Geometry: final body of the model. Coordinates: model frame, mm. Face numbers are marked on the shaded views. A direction names the side the tool comes from. Coordinates: 2 decimals unless noted, no trailing zeros. Loops run counter-clockwise (first coordinate to the right, second up) from the corner with the lowest first, then second, coordinate; pieces in that order, holes last. Notation, with made-up numbers: (-17.5, -0.75) -> (-7.5, -0.75) arc R21 ccw to (-7.5, 8.25) -> close; hole circle Ø11 at (55.5, -40). An arc over 180 degrees is marked (long way). One line per item, written item: value. Start each with the question number.
from build123d import *

# Parameters (mm, degrees)
SKETCH1_W           = 180
SKETCH1_H           = 200
BOSS_EXTRUDE1_DEPTH = 12.5
SKETCH2_W           = 85
SKETCH2_H           = 55
CUT_EXTRUDE1_DEPTH  = 1.5
SKETCH3_W           = 105
SKETCH3_H           = 35
CUT_EXTRUDE2_DEPTH  = 1.5
SKETCH4_W           = 180
SKETCH4_H           = 200
CUT_EXTRUDE3_DEPTH  = 4.5
SKETCH5_W           = 180
SKETCH5_H           = 200
CUT_EXTRUDE4_DEPTH  = 3
SKETCH7_W           = 85
SKETCH7_H           = 55
BOSS_EXTRUDE2_DEPTH = 1.5
SKETCH8_W           = 50
SKETCH8_H           = 50
CUT_EXTRUDE5_DEPTH  = 1.5
SKETCH9_W           = 66
SKETCH9_H           = 36
CUT_EXTRUDE6_DEPTH  = 1.5
SKETCH11_W          = 80
SKETCH11_H          = 40
SKETCH11_W_2        = 97
SKETCH11_H_2        = 20
CUT_EXTRUDE9_DEPTH  = 1.5
SKETCH15_R          = 1.35
CUT_EXTRUDE11_DEPTH = 135.629120178
SKETCH16_R          = 1.75
CUT_EXTRUDE12_DEPTH = 5


with BuildPart() as part:
    # Sketch1 → Boss-Extrude1 (new body)
    with BuildSketch(Plane(origin=(0, 0, 0), x_dir=(1, 0, 0), z_dir=(0, 1, 0))):
        Rectangle(SKETCH1_W, SKETCH1_H)
    extrude(amount=BOSS_EXTRUDE1_DEPTH)

    # Sketch2 → Cut-Extrude1 (cut)
    with BuildSketch(Plane(origin=(0, 12.5, 0), x_dir=(1, 0, 0), z_dir=(0, 1, 0))):
        Rectangle(SKETCH2_W, SKETCH2_H)
    extrude(amount=-CUT_EXTRUDE1_DEPTH, mode=Mode.SUBTRACT)

    # Sketch3 → Cut-Extrude2 (cut)
    with BuildSketch(Plane(origin=(0, 12.5, 0), x_dir=(1, 0, 0), z_dir=(0, 1, 0))):
        with Locations((0, 67.5)):
            Rectangle(SKETCH3_W, SKETCH3_H)
    extrude(amount=-CUT_EXTRUDE2_DEPTH, mode=Mode.SUBTRACT)

    # Sketch4 → Cut-Extrude3 (cut)
    with BuildSketch(Plane.XZ):
        Rectangle(SKETCH4_W, SKETCH4_H)
    extrude(amount=-CUT_EXTRUDE3_DEPTH, mode=Mode.SUBTRACT)

    # Sketch5 → Cut-Extrude4 (cut)
    with BuildSketch(Plane.XZ.offset(-4.5)):
        Rectangle(SKETCH5_W, SKETCH5_H)
    extrude(amount=-CUT_EXTRUDE4_DEPTH, mode=Mode.SUBTRACT)

    # Sketch7 → Boss-Extrude2 (add)
    with BuildSketch(Plane(origin=(0, 11, 0), x_dir=(1, 0, 0), z_dir=(0, 1, 0))):
        Rectangle(SKETCH7_W, SKETCH7_H)
    extrude(amount=BOSS_EXTRUDE2_DEPTH)

    # Sketch8 → Cut-Extrude5 (cut)
    with BuildSketch(Plane(origin=(0, 12.5, 0), x_dir=(1, 0, 0), z_dir=(0, 1, 0))):
        with Locations((55, 0)):
            Rectangle(SKETCH8_W, SKETCH8_H)
        with Locations((-55, 0)):
            Rectangle(SKETCH8_W, SKETCH8_H)
    extrude(amount=-CUT_EXTRUDE5_DEPTH, mode=Mode.SUBTRACT)

    # Sketch9 → Cut-Extrude6 (cut)
    with BuildSketch(Plane(origin=(0, 12.5, 0), x_dir=(1, 0, 0), z_dir=(0, 1, 0))):
        with Locations((44.314846592, -53.31046024)):
            Rectangle(SKETCH9_W, SKETCH9_H)
        with Locations((-44.314846592, -53.31046024)):
            Rectangle(SKETCH9_W, SKETCH9_H)
    extrude(amount=-CUT_EXTRUDE6_DEPTH, mode=Mode.SUBTRACT)

    # Sketch11 → Cut-Extrude9 (cut)
    with BuildSketch(Plane.XZ.offset(-7.5)):
        with Locations((-90, 43.788146999)):
            Rectangle(SKETCH11_W, SKETCH11_H)
        with Locations((-90, -61.211853001)):
            Rectangle(SKETCH11_W, SKETCH11_H)
        with Locations((90, -60)):
            Rectangle(SKETCH11_W, SKETCH11_H)
        with Locations((0, 89.411235459)):
            Rectangle(SKETCH11_W_2, SKETCH11_H_2)
        with Locations((90, 43.788146999)):
            Rectangle(SKETCH11_W, SKETCH11_H)
    extrude(amount=-CUT_EXTRUDE9_DEPTH, mode=Mode.SUBTRACT)

    # Sketch15 → Cut-Extrude11 (cut, through all)
    with BuildSketch(Plane.XZ.offset(-7.5)):
        with Locations(Location((-20, 25, 0), (0, 0, 270))):
            Circle(SKETCH15_R)
        with Locations(Location((20, 25, 0), (0, 0, 270))):
            Circle(SKETCH15_R)
        with Locations(Location((-20, -35, 0), (0, 0, 270))):
            Circle(SKETCH15_R)
        with Locations(Location((20, -35, 0), (0, 0, 270))):
            Circle(SKETCH15_R)
    extrude(amount=-CUT_EXTRUDE11_DEPTH, mode=Mode.SUBTRACT)

    # Sketch16 → Cut-Extrude12 (cut)
    with BuildSketch(Plane(origin=(0, 12.5, 0), x_dir=(1, 0, 0), z_dir=(0, 1, 0))):
        with Locations(Location((-75, -85, 0), (0, 0, 270))):
            Circle(SKETCH16_R)
        with Locations(Location((75, -85, 0), (0, 0, 90))):
            Circle(SKETCH16_R)
    extrude(amount=-CUT_EXTRUDE12_DEPTH, mode=Mode.SUBTRACT)


solid = part.part
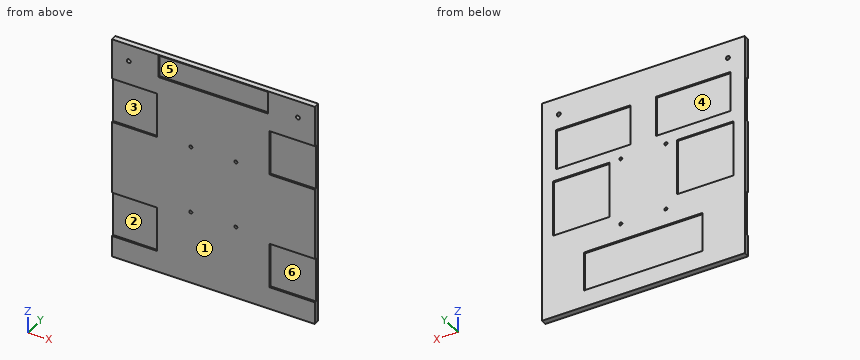
1. Line query: L1, parallel to X at y = 8.55, z = 25; L2, parallel to X at y = 11.3, z = -35; L3, parallel to X at y = 12.3, z = -63.5. Output: solid intervals per line, ascending. Write a range as [from, to].
2. Pin query (flat end, axial travel): pin 1 Ø20 at (x, z) = (67, 47.5) entering from -Y; pin 2 Ø1.6 at (x, z) = (20, -35) entering from -Y (3 decimals). Return the tip coordinate at first contact, or that it passes through.
3. Set-up query: the marked faces 3, 4, 5 and 6. Return all of +Z, -Z, +X, -X, +Y, -Y with unobstructed straight access to the full face (end or side cutting, diameter ignored); none if empty.
4. Section A-A on x = 4. Return the cut outline in (y, z), plus the area to 4 significant figures.
5. Draft query along Z for the marked faces 1 and 2. Return one class per face: released by +Z, released by -Z, zero draft, split by the parting line, or undercut.
6. Section B-B on z = -21.5. Return the cut outline in (x, y).
7. Section C-C on x = -70. Return the cut outline in (y, z).
Checks:
1. L1: [-50, -21.35], [-18.65, 18.65], [21.35, 50]
1. L2: [-90, -21.35], [-18.65, 18.65], [21.35, 90]
1. L3: [-90, -52.5], [52.5, 90]
2. pin 1: y = 9
2. pin 2: through
3. face 3: -X, -Y
3. face 4: +Y
3. face 5: -Y
3. face 6: +X, -Y
4. outline: (7.5, -100) -> (12.5, -100) -> (12.5, -85) -> (11, -85) -> (11, -50) -> (12.5, -50) -> (12.5, 100) -> (7.5, 100) -> (7.5, 99.41) -> (9, 99.41) -> (9, 79.41) -> (7.5, 79.41) -> close
4. area: 917.5 mm²
5. face 1: zero draft
5. face 2: undercut
6. outline: (-90, 7.5) -> (90, 7.5) -> (90, 12.5) -> (80, 12.5) -> (80, 11) -> (30, 11) -> (30, 12.5) -> (-30, 12.5) -> (-30, 11) -> (-80, 11) -> (-80, 12.5) -> (-90, 12.5) -> close
7. outline: (7.5, -100) -> (12.5, -100) -> (12.5, -25) -> (11, -25) -> (11, 25) -> (12.5, 25) -> (12.5, 35.31) -> (11, 35.31) -> (11, 71.31) -> (12.5, 71.31) -> (12.5, 100) -> (7.5, 100) -> (7.5, 63.79) -> (9, 63.79) -> (9, 23.79) -> (7.5, 23.79) -> (7.5, -41.21) -> (9, -41.21) -> (9, -81.21) -> (7.5, -81.21) -> close
